Check sheet for the drawn part. Datum: minimum x, y, z corner. Units: mm. A direction names the side the tool comes from. Coordinates: 2 decimals unless noted, no trailing zeros. Loops run counter-clockwise (first coordinate to the right, second up) from the corner with the lowest first, then second, coordinate; pieces in that order, holes last.
Q1. Go/stop test with flat-tipped pins: P1, Ø4.5, axis at x = 4, z = 4.5, coming from the -Y side; P2, Ø7, axis at x = 5.5, y = 17, coming from the +Z side; P3, Ø8, axis at x = 10, z = 39.5, coming from the +Y side; P4, Ø7, axis at x = 2.5, y = 60.5, coming from the -Z side. Record where each tip stops, or that it passes through.
Q2. Access from +Z, -Z, +X, -X, +Y, -Y to the whole of each face (thin tool, end or side, straight path). Record for the marked faces 4, 5, 6 and 7.
Q3. Sectioned sample at D-D (y = 62.5). Enter the section's corners in (x, z).
Q4. Sectioned sample at A-A (z = 49). Enter the section's corners in (x, y).
Q5. Material ranges on probe 1 along Z at (x, y) = (7, 11); probe 2 along X at (y, z) = (31.5, 72); probe 3 along Z at (x, y) = (3, 3), recorded low to high.
Q6. Mould release check, pull along Z, two halves, no side actions. Record for the marked faces 1, 2 and 3: +Z half, -Z half, draft (parallel to the pull), parting line (faces both ways), or undercut.
Q7. Sectioned sample at B-B (y = 35). Enter the section's corners in (x, z), then the cut area to 3 significant figures.
Q8. Sectioned sample at C-C (x = 6). Enter the section's corners in (y, z), then the cut area to 3 significant figures.
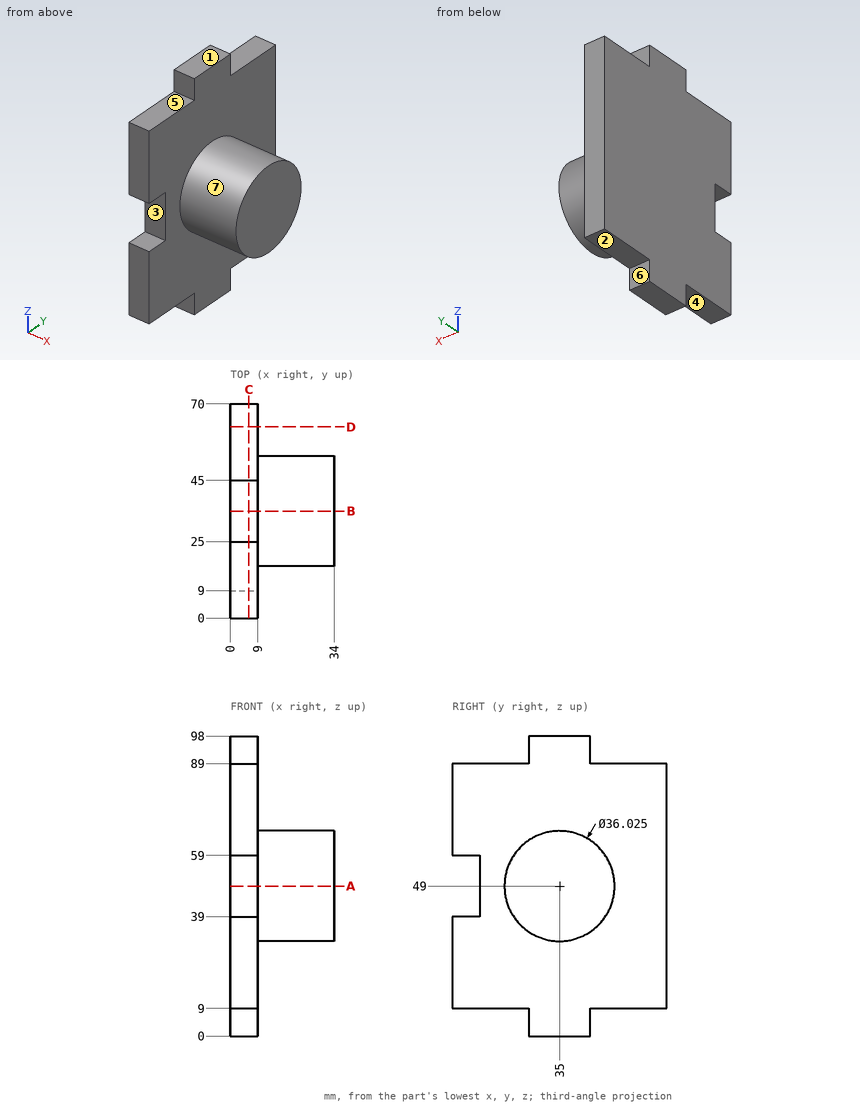
Geometry check:
1. P1: stops at y = 25
1. P2: stops at z = 89
1. P3: stops at y = 70
1. P4: stops at z = 9
2. face 4: -Z, +X, -X, -Y
2. face 5: +Z, +X, -X, -Y
2. face 6: -Z, +X, -X, +Y
2. face 7: +X
3. outline: (0, 9) - (9, 9) - (9, 89) - (0, 89) - close
4. outline: (0, 9) - (9, 9) - (9, 16.99) - (34, 16.99) - (34, 53.01) - (9, 53.01) - (9, 70) - (0, 70) - close
5. probe 1: z = 9 to 89
5. probe 2: x = 0 to 9
5. probe 3: z = 9 to 39, 59 to 89
6. face 1: +Z half
6. face 2: -Z half
6. face 3: undercut
7. outline: (0, 0) - (9, 0) - (9, 30.99) - (34, 30.99) - (34, 67.01) - (9, 67.01) - (9, 98) - (0, 98) - close
7. area: 1,780 mm2
8. outline: (0, 9) - (25, 9) - (25, 0) - (45, 0) - (45, 9) - (70, 9) - (70, 89) - (45, 89) - (45, 98) - (25, 98) - (25, 89) - (0, 89) - (0, 59) - (9, 59) - (9, 39) - (0, 39) - close
8. area: 5,780 mm2
